Geometry check sheet. Reference: drawing and pictorial views, mm from the part's lowest x, y, z. A direction names the side the tool comes from. Give positions to 0.01 mm unless a question says otherwise; leave off trailing zeros. Order: outer loops, then holes, each group sorted by start corner. A loop starts at its lowest first (then second) coordinate and runs counter-clockwise, first axis right, second up. Notation, with made-up numbers: M -19,16 L 29,16 A15 ccw 29,21 Z; hole C 25,67.25 d8. An arc over 180 degrees is marked long. Answer as a JSON object with one key per item and string values. Group by question number.
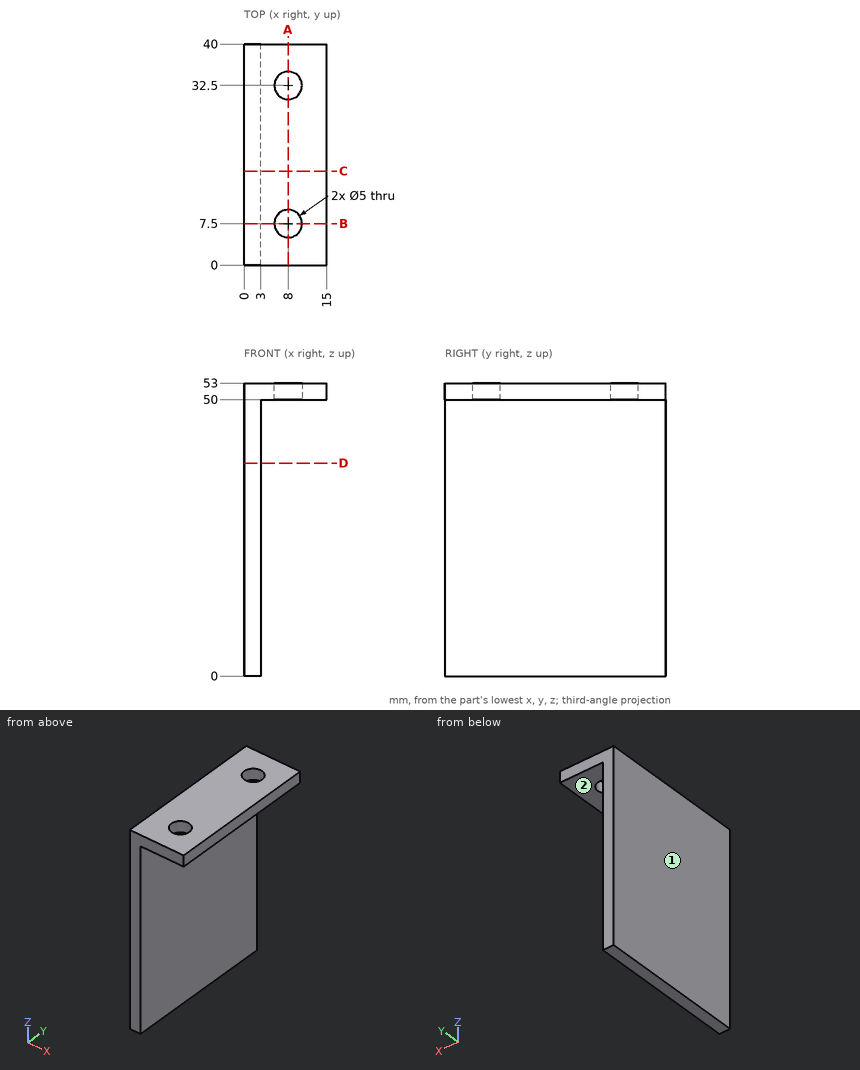
1. Cross-section at B-B (y = 7.5). Record the cut outline in (x, z).
2. Depth check by flat-ended pin: pin 1 (12 mm diameter, centred on y = 15, z = 11, fed in from -X); pin 2 (1.5 mm diameter, centred on x = 8.5, y = 27.5, fed in from -Z). Enter the tip coordinate at first touch or a pass-through.
3. Thickness scan on line 1 along Y through (x, z) = (8, 52.3); line 2 along Z through (x, y) = (10.5, 12); line 3 along X through (y, z) = (5, 4.5). Record the ranges inside material, lowest first. Write a range as [from, to].
4. Cross-section at C-C (y = 17). Record the cut outline in (x, z), and give its area (3 significant figures).
5. Cross-section at A-A (x = 8). Record the cut outline in (y, z).
6. Access from +Z, -Z, +X, -X, +Y, -Y to the whole of each face (thin tool, end or side, straight path). Record for the marked faces 1 and 2.
7. Cross-section at D-D (z = 38.5). Record the cut outline in (x, y).
Report:
{
 "1": {"outline": "M 0,0 L 3,0 L 3,50 L 5.5,50 L 5.5,53 L 0,53 Z; M 10.5,50 L 15,50 L 15,53 L 10.5,53 Z"},
 "2": {"pin 1": "stops at x = 0", "pin 2": "stops at z = 50"},
 "3": {"line 1": "y = [0, 5], [10, 30], [35, 40]", "line 2": "z = [50, 53]", "line 3": "x = [0, 3]"},
 "4": {"outline": "M 0,0 L 3,0 L 3,50 L 15,50 L 15,53 L 0,53 Z", "area": "195 mm2"},
 "5": {"outline": "M 0,50 L 5,50 L 5,53 L 0,53 Z; M 10,50 L 30,50 L 30,53 L 10,53 Z; M 35,50 L 40,50 L 40,53 L 35,53 Z"},
 "6": {"face 1": "+Z, -Z, -X, +Y, -Y", "face 2": "-Z, +X, +Y, -Y"},
 "7": {"outline": "M 0,0 L 3,0 L 3,40 L 0,40 Z"}
}
